from build123d import *

# Parameters (mm, degrees)
SKETCH1_R           = 1.675
BOSS_EXTRUDE1_DEPTH = 3
SKETCH2_R           = 1.675
BOSS_EXTRUDE2_DEPTH = 3


with BuildPart() as part:
    # Sketch1 → Boss-Extrude1 (new body)
    with BuildSketch(Plane(origin=(3, 0, 0), x_dir=(0, 0, -1), z_dir=(1, 0, 0))):
        with BuildLine():
            ThreePointArc((-14.537314892, 1.599093719), (-13.375367565, 0.916420874), (-12.080565177, 0.542722358))
            ThreePointArc((-12.080565177, 0.542722358), (-12.09275, 0), (-12.080565177, -0.542722358))
            ThreePointArc((-12.080565177, -0.542722358), (-13.375367565, -0.916420874), (-14.537314892, -1.599093719))
            ThreePointArc((-14.537314892, -1.599093719), (-14.499881098, -1.908945561), (-14.455843809, -2.217928037))
            ThreePointArc((-14.455843809, -2.217928037), (-13.156800143, -2.576605271), (-11.809396783, -2.602450802))
            ThreePointArc((-11.809396783, -2.602450802), (-11.680699536, -3.129834008), (-11.528463019, -3.650909885))
            ThreePointArc((-11.528463019, -3.650909885), (-12.682425791, -4.346994451), (-13.62809199, -5.30713988))
            ThreePointArc((-13.62809199, -5.30713988), (-13.511738163, -5.596745198), (-13.389230859, -5.883801663))
            ThreePointArc((-13.389230859, -5.883801663), (-12.041618533, -5.894040025), (-10.733437515, -5.57027124))
            ThreePointArc((-10.733437515, -5.57027124), (-10.472628702, -6.046375), (-10.190715157, -6.510293938))
            ThreePointArc((-10.190715157, -6.510293938), (-11.125197659, -7.48132754), (-11.79013714, -8.65351323))
            ThreePointArc((-11.79013714, -8.65351323), (-11.602792602, -8.903135899), (-11.410163953, -9.148703928))
            ThreePointArc((-11.410163953, -9.148703928), (-10.105820521, -8.809805691), (-8.926012217, -8.158486898))
            ThreePointArc((-8.926012217, -8.158486898), (-8.550865528, -8.550865528), (-8.158486898, -8.926012217))
            ThreePointArc((-8.158486898, -8.926012217), (-8.809805691, -10.105820521), (-9.148703928, -11.410163953))
            ThreePointArc((-9.148703928, -11.410163953), (-8.903135899, -11.602792602), (-8.65351323, -11.79013714))
            ThreePointArc((-8.65351323, -11.79013714), (-7.48132754, -11.125197659), (-6.510293938, -10.190715157))
            ThreePointArc((-6.510293938, -10.190715157), (-6.046375, -10.472628702), (-5.57027124, -10.733437515))
            ThreePointArc((-5.57027124, -10.733437515), (-5.894040025, -12.041618533), (-5.883801663, -13.389230859))
            ThreePointArc((-5.883801663, -13.389230859), (-5.596745198, -13.511738163), (-5.30713988, -13.62809199))
            ThreePointArc((-5.30713988, -13.62809199), (-4.346994451, -12.682425791), (-3.650909885, -11.528463019))
            ThreePointArc((-3.650909885, -11.528463019), (-3.129834008, -11.680699536), (-2.602450802, -11.809396783))
            ThreePointArc((-2.602450802, -11.809396783), (-2.576605271, -13.156800143), (-2.217928037, -14.455843809))
            ThreePointArc((-2.217928037, -14.455843809), (-1.908945561, -14.499881098), (-1.599093719, -14.537314892))
            ThreePointArc((-1.599093719, -14.537314892), (-0.916420874, -13.375367565), (-0.542722358, -12.080565177))
            ThreePointArc((-0.542722358, -12.080565177), (0, -12.09275), (0.542722358, -12.080565177))
            ThreePointArc((0.542722358, -12.080565177), (0.916420874, -13.375367565), (1.599093719, -14.537314892))
            ThreePointArc((1.599093719, -14.537314892), (1.908945561, -14.499881098), (2.217928037, -14.455843809))
            ThreePointArc((2.217928037, -14.455843809), (2.576605271, -13.156800143), (2.602450802, -11.809396783))
            ThreePointArc((2.602450802, -11.809396783), (3.129834008, -11.680699536), (3.650909885, -11.528463019))
            ThreePointArc((3.650909885, -11.528463019), (4.346994451, -12.682425791), (5.30713988, -13.62809199))
            ThreePointArc((5.30713988, -13.62809199), (5.596745198, -13.511738163), (5.883801663, -13.389230859))
            ThreePointArc((5.883801663, -13.389230859), (5.894040025, -12.041618533), (5.57027124, -10.733437515))
            ThreePointArc((5.57027124, -10.733437515), (6.046375, -10.472628702), (6.510293938, -10.190715157))
            ThreePointArc((6.510293938, -10.190715157), (7.48132754, -11.125197659), (8.65351323, -11.79013714))
            ThreePointArc((8.65351323, -11.79013714), (8.903135899, -11.602792602), (9.148703928, -11.410163953))
            ThreePointArc((9.148703928, -11.410163953), (8.809805691, -10.105820521), (8.158486898, -8.926012217))
            ThreePointArc((8.158486898, -8.926012217), (8.550865528, -8.550865528), (8.926012217, -8.158486898))
            ThreePointArc((8.926012217, -8.158486898), (10.105820521, -8.809805691), (11.410163953, -9.148703928))
            ThreePointArc((11.410163953, -9.148703928), (11.602792602, -8.903135899), (11.79013714, -8.65351323))
            ThreePointArc((11.79013714, -8.65351323), (11.125197659, -7.48132754), (10.190715157, -6.510293938))
            ThreePointArc((10.190715157, -6.510293938), (10.472628702, -6.046375), (10.733437515, -5.57027124))
            ThreePointArc((10.733437515, -5.57027124), (12.041618533, -5.894040025), (13.389230859, -5.883801663))
            ThreePointArc((13.389230859, -5.883801663), (13.511738163, -5.596745198), (13.62809199, -5.30713988))
            ThreePointArc((13.62809199, -5.30713988), (12.682425791, -4.346994451), (11.528463019, -3.650909885))
            ThreePointArc((11.528463019, -3.650909885), (11.680699536, -3.129834008), (11.809396783, -2.602450802))
            ThreePointArc((11.809396783, -2.602450802), (13.156800143, -2.576605271), (14.455843809, -2.217928037))
            ThreePointArc((14.455843809, -2.217928037), (14.499881098, -1.908945561), (14.537314892, -1.599093719))
            ThreePointArc((14.537314892, -1.599093719), (13.375367565, -0.916420874), (12.080565177, -0.542722358))
            ThreePointArc((12.080565177, -0.542722358), (12.09275, 0), (12.080565177, 0.542722358))
            ThreePointArc((12.080565177, 0.542722358), (13.375367565, 0.916420874), (14.537314892, 1.599093719))
            ThreePointArc((14.537314892, 1.599093719), (14.499881098, 1.908945561), (14.455843809, 2.217928037))
            ThreePointArc((14.455843809, 2.217928037), (13.156800143, 2.576605271), (11.809396783, 2.602450802))
            ThreePointArc((11.809396783, 2.602450802), (11.680699536, 3.129834008), (11.528463019, 3.650909885))
            ThreePointArc((11.528463019, 3.650909885), (12.682425791, 4.346994451), (13.62809199, 5.30713988))
            ThreePointArc((13.62809199, 5.30713988), (13.511738163, 5.596745198), (13.389230859, 5.883801663))
            ThreePointArc((13.389230859, 5.883801663), (12.041618533, 5.894040025), (10.733437515, 5.57027124))
            ThreePointArc((10.733437515, 5.57027124), (10.472628702, 6.046375), (10.190715157, 6.510293938))
            ThreePointArc((10.190715157, 6.510293938), (11.125197659, 7.48132754), (11.79013714, 8.65351323))
            ThreePointArc((11.79013714, 8.65351323), (11.602792602, 8.903135899), (11.410163953, 9.148703928))
            ThreePointArc((11.410163953, 9.148703928), (10.105820521, 8.809805691), (8.926012217, 8.158486898))
            ThreePointArc((8.926012217, 8.158486898), (8.550865528, 8.550865528), (8.158486898, 8.926012217))
            ThreePointArc((8.158486898, 8.926012217), (8.809805691, 10.105820521), (9.148703928, 11.410163953))
            ThreePointArc((9.148703928, 11.410163953), (8.903135899, 11.602792602), (8.65351323, 11.79013714))
            ThreePointArc((8.65351323, 11.79013714), (7.48132754, 11.125197659), (6.510293938, 10.190715157))
            ThreePointArc((6.510293938, 10.190715157), (6.046375, 10.472628702), (5.57027124, 10.733437515))
            ThreePointArc((5.57027124, 10.733437515), (5.894040025, 12.041618533), (5.883801663, 13.389230859))
            ThreePointArc((5.883801663, 13.389230859), (5.596745198, 13.511738163), (5.30713988, 13.62809199))
            ThreePointArc((5.30713988, 13.62809199), (4.346994451, 12.682425791), (3.650909885, 11.528463019))
            ThreePointArc((3.650909885, 11.528463019), (3.129834008, 11.680699536), (2.602450802, 11.809396783))
            ThreePointArc((2.602450802, 11.809396783), (2.576605271, 13.156800143), (2.217928037, 14.455843809))
            ThreePointArc((2.217928037, 14.455843809), (1.908945561, 14.499881098), (1.599093719, 14.537314892))
            ThreePointArc((1.599093719, 14.537314892), (0.916420874, 13.375367565), (0.542722358, 12.080565177))
            ThreePointArc((0.542722358, 12.080565177), (0, 12.09275), (-0.542722358, 12.080565177))
            ThreePointArc((-0.542722358, 12.080565177), (-0.916420874, 13.375367565), (-1.599093719, 14.537314892))
            ThreePointArc((-1.599093719, 14.537314892), (-1.908945561, 14.499881098), (-2.217928037, 14.455843809))
            ThreePointArc((-2.217928037, 14.455843809), (-2.576605271, 13.156800143), (-2.602450802, 11.809396783))
            ThreePointArc((-2.602450802, 11.809396783), (-3.129834008, 11.680699536), (-3.650909885, 11.528463019))
            ThreePointArc((-3.650909885, 11.528463019), (-4.346994451, 12.682425791), (-5.30713988, 13.62809199))
            ThreePointArc((-5.30713988, 13.62809199), (-5.596745198, 13.511738163), (-5.883801663, 13.389230859))
            ThreePointArc((-5.883801663, 13.389230859), (-5.894040025, 12.041618533), (-5.57027124, 10.733437515))
            ThreePointArc((-5.57027124, 10.733437515), (-6.046375, 10.472628702), (-6.510293938, 10.190715157))
            ThreePointArc((-6.510293938, 10.190715157), (-7.48132754, 11.125197659), (-8.65351323, 11.79013714))
            ThreePointArc((-8.65351323, 11.79013714), (-8.903135899, 11.602792602), (-9.148703928, 11.410163953))
            ThreePointArc((-9.148703928, 11.410163953), (-8.809805691, 10.105820521), (-8.158486898, 8.926012217))
            ThreePointArc((-8.158486898, 8.926012217), (-8.550865528, 8.550865528), (-8.926012217, 8.158486898))
            ThreePointArc((-8.926012217, 8.158486898), (-10.105820521, 8.809805691), (-11.410163953, 9.148703928))
            ThreePointArc((-11.410163953, 9.148703928), (-11.602792602, 8.903135899), (-11.79013714, 8.65351323))
            ThreePointArc((-11.79013714, 8.65351323), (-11.125197659, 7.48132754), (-10.190715157, 6.510293938))
            ThreePointArc((-10.190715157, 6.510293938), (-10.472628702, 6.046375), (-10.733437515, 5.57027124))
            ThreePointArc((-10.733437515, 5.57027124), (-12.041618533, 5.894040025), (-13.389230859, 5.883801663))
            ThreePointArc((-13.389230859, 5.883801663), (-13.511738163, 5.596745198), (-13.62809199, 5.30713988))
            ThreePointArc((-13.62809199, 5.30713988), (-12.682425791, 4.346994451), (-11.528463019, 3.650909885))
            ThreePointArc((-11.528463019, 3.650909885), (-11.680699536, 3.129834008), (-11.809396783, 2.602450802))
            ThreePointArc((-11.809396783, 2.602450802), (-13.156800143, 2.576605271), (-14.455843809, 2.217928037))
            ThreePointArc((-14.455843809, 2.217928037), (-14.499881098, 1.908945561), (-14.537314892, 1.599093719))
        make_face()
        with Locations(Location((0, 0, 0), (0, 0, 180))):
            Circle(SKETCH1_R, mode=Mode.SUBTRACT)
    extrude(amount=-BOSS_EXTRUDE1_DEPTH)

    # Sketch2 → Boss-Extrude2 (add)
    with BuildSketch(Plane(origin=(3, 0, 0), x_dir=(0, 0, -1), z_dir=(1, 0, 0))):
        with BuildLine():
            Line((0, -4), (-31, -4))
            ThreePointArc((-31, -4), (-35, 0), (-31, 4))
            Line((-31, 4), (0, 4))
            ThreePointArc((0, 4), (4, 0), (0, -4))
        make_face()
        with Locations((-31, 0)):
            Circle(SKETCH2_R, mode=Mode.SUBTRACT)
        with Locations(Location((0, 0, 0), (0, 0, 180))):
            Circle(SKETCH2_R, mode=Mode.SUBTRACT)
    extrude(amount=-BOSS_EXTRUDE2_DEPTH)


solid = part.part
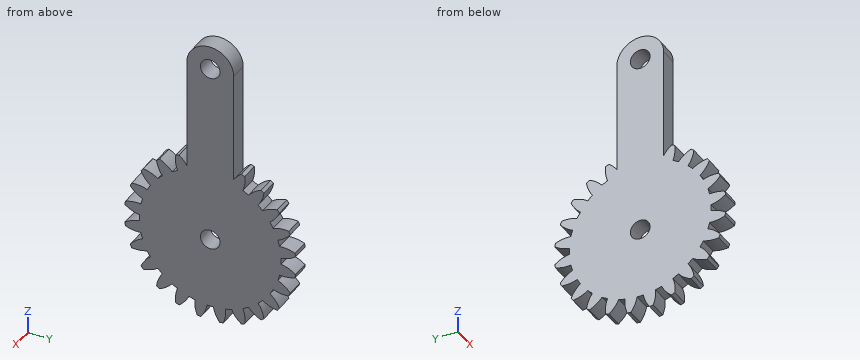
Geometry check sheet. Reference: the model listing, model coordinates, mm. Round coordinates to 2 decimals unless told otherwise and drop trailing zeros. Order: outer loops, then holes, each group sorted by start corner. A loop starts at its lowest first (then second) coordinate and runs counter-clockwise, first axis right, second up. Notation, with made-up numbers: (-32, 30) - (-8, 30) arc R21 ccw to (-8, 46) - close; hole circle Ø11 at (80, 79.5). An arc over 180 degrees is marked (long way). One line per question, with ' | ' between items. Start each with the question number.
(1) Sectioned sample at B-B on y = 0. Record the cut outline in (x, z) (3 decimals).
(2) Sectioned sample at C-C on y = -12.75. Record the cut outline in (x, z), and give its area (3 significant figures).
(3) Sectioned sample at A-A on z = 0. Record the cut outline in (x, y) (3 decimals), and give its area (3 significant figures).
(4) Depth check by flat-ended pin: pin 1 Ø4 at (y, z) = (0, 0) entering from +X; pin 2 Ø1.5 at (x, z) = (2, 11.5) entering from -Y; pin 3 Ø2 at (y, z) = (0, 31) entering from -X. Enter the tip coordinate at first touch or a pass-through.
(5) Thickness scan on L1, parallel to Y at x = 2.1, z = 0 (3 decimals); L2, parallel to Y at x = 1.1, z = 31 (3 decimals); L3, parallel to Z at x = 1.8, y = 0.5. Record the ranges inside material, lowest first. Write a range as [from, to].
(6) Sectioned sample at D-D on x = 1.2. Count the separate pieces of the cut face and the enclosed holes in it, and give its area (3 significant figures).
Conclusion:
1) outline: (0, -12.093) - (3, -12.093) - (3, -1.675) - (0, -1.675) - close; (0, 1.675) - (3, 1.675) - (3, 29.325) - (0, 29.325) - close; (0, 32.675) - (3, 32.675) - (3, 35) - (0, 35) - close
2) outline: (0, -5.93) - (3, -5.93) - (3, -4.4) - (0, -4.4) - close; (0, -2.62) - (3, -2.62) - (3, -0.69) - (0, -0.69) - close; (0, 0.69) - (3, 0.69) - (3, 2.62) - (0, 2.62) - close; (0, 4.4) - (3, 4.4) - (3, 5.93) - (0, 5.93) - close | area: 20.7 mm2
3) outline: (0, -12.093) - (3, -12.093) - (3, -1.675) - (0, -1.675) - close; (0, 1.675) - (3, 1.675) - (3, 12.093) - (0, 12.093) - close | area: 62.5 mm2
4) pin 1: stops at x = 3 | pin 2: stops at y = -9.15 | pin 3: passes through
5) L1: y = [-12.093, -1.675], [1.675, 12.093] | L2: y = [-4, -1.675], [1.675, 4] | L3: z = [-12.08, -1.6], [1.6, 29.4], [32.6, 34.97]
6) separate pieces: 1 | enclosed holes: 2 | area: 708 mm2
